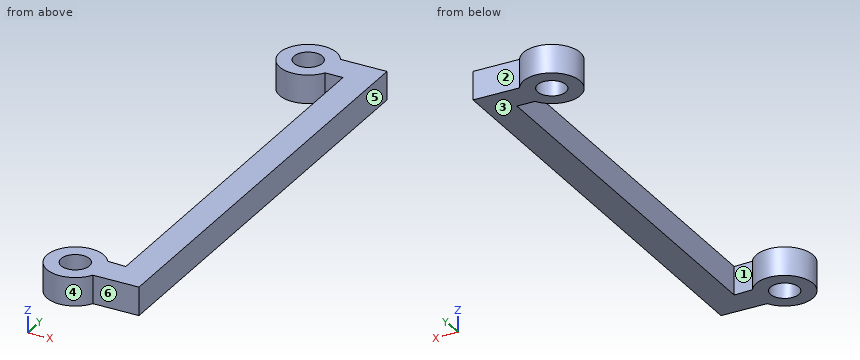
from build123d import *

# Parameters (mm, degrees)
SKETCH_R      = 10
EXTRUDE_DEPTH = 20


with BuildPart() as part:
    # Sketch → Extrude (new body)
    with BuildSketch(Plane.XY):
        with BuildLine():
            Line((11.677619, 0.722876), (24.795086, 0))
            Line((24.795086, 280), (24.795086, 0))
            Line((24.795086, 280), (12.115594, 280))
            ThreePointArc((12.115594, 300), (-25.204914, 290), (12.115594, 280))
            Line((12.115594, 300), (44.795086, 300))
            Line((44.795086, 300), (44.795086, -19.596431))
            Line((44.795086, -19.596431), (12.342408, -19.596431))
            ThreePointArc((11.677619, 0.722876), (-25.194218, -10.653992), (12.342408, -19.596431))
        make_face()
        with Locations((-5.204914, -10)):
            Circle(SKETCH_R, mode=Mode.SUBTRACT)
        with Locations((-5.204914, 290)):
            Circle(SKETCH_R, mode=Mode.SUBTRACT)
    extrude(amount=EXTRUDE_DEPTH)


solid = part.part
The listing builds one solid part. Answer for the finished solid, in the listing's coordinates (mm). Face numbers are marked on the shaded views. A direction names the side the tool comes from. Round coordinates to 2 decimals unless told otherwise and drop trailing zeros. Order: outer loops, then holes, each group sorted by start corner. A loop starts at its lowest first (then second) coordinate and runs counter-clockwise, first axis right, second up. Notation, with made-up numbers: (84, 18.25) - (115, 18.25) arc R22 ccw to (115, 55.25) - close; hole circle Ø11 at (-6, -2). An arc over 180 degrees is marked (long way). Write item = value, one per line. Start each with the question number.
1) Section C-C, the plane x = -2 is taken. Write down the section's boundary in (y, z), plus the area to 3 significant figures.
2) Section D-D, the plane x = 16.5 is taken. Write down the section's boundary in (y, z).
3) For the marked faces 1, 2 and 3, determine the directions among +Z, -Z, +X, -X, +Y, -Y from which every point of the face is accessible in a straight line to the end or side of a thin tool.
4) For a pull along Y with two mould halves and no side action, classify the marked faces 4, 5 and 6 as released by +Y, released by -Y, zero draft, split by the parting line, or undercut.
5) Given pin 1 (8 mm diameter, centred on x = 2, z = 17, fed in from +Y); pin 2 (6 mm diameter, centred on x = -10.5, z = 5.5, fed in from +Y); pin 3 (6 mm diameter, centred on x = 33.5, z = 8, fed in from +Y); pin 4 (12 mm diameter, centred on x = -5.2, y = 290, fed in from +Z), each flat-ended and moving along its own axis, determine where each tip first touches the part or whether it passes through.
6) Straight lines are drawn through the part: L1, parallel to Y at x = -12.5, z = 5; L2, parallel to Y at x = -10, z = 3.5; L3, parallel to X at y = 237, z = 15.25. For each, find the intervals that lie inside material, in ascending order.
7) Section B-B, the plane y = 290 is taken. Write down the section's boundary in (x, z), plus the area to 3 significant figures.
8) Section A-A, the plane z = 3.5 is taken. Write down the section's boundary in (x, y), plus the area to 3 significant figures.
Results list:
q1.outline = (-29.74, 0) - (-19.47, 0) - (-19.47, 20) - (-29.74, 20) - close; (-0.53, 0) - (9.74, 0) - (9.74, 20) - (-0.53, 20) - close; (270.26, 0) - (280.53, 0) - (280.53, 20) - (270.26, 20) - close; (299.47, 0) - (309.74, 0) - (309.74, 20) - (299.47, 20) - close
q1.area = 822 mm^2
q2.outline = (-19.6, 0) - (0.46, 0) - (0.46, 20) - (-19.6, 20) - close; (280, 0) - (300, 0) - (300, 20) - (280, 20) - close
q3.face_1 = +Z, -Z
q3.face_2 = +Z, -Z, +X, +Y
q3.face_3 = -Z, +X, -X, +Y, -Y
q4.face_4 = undercut
q4.face_5 = zero draft
q4.face_6 = released by -Y
q5.pin_1 = 309.74
q5.pin_2 = 309.87
q5.pin_3 = 300
q5.pin_4 = through
q6.L1 = -28.62 to -16.84, -3.16 to 8.62, 271.38 to 283.16, 296.84 to 308.62
q6.L2 = -29.42 to -18.78, -1.22 to 9.42, 270.58 to 281.22, 298.78 to 309.42
q6.L3 = 24.8 to 44.8
q7.outline = (-25.2, 0) - (-15.2, 0) - (-15.2, 20) - (-25.2, 20) - close; (4.8, 0) - (44.8, 0) - (44.8, 20) - (4.8, 20) - close
q7.area = 1,000 mm^2
q8.outline = (11.68, 0.72) arc R20 ccw (long way) to (12.34, -19.6) - (44.8, -19.6) - (44.8, 300) - (12.12, 300) arc R20 ccw (long way) to (12.12, 280) - (24.8, 280) - (24.8, 0) - close; hole circle Ø20 at (-5.2, -10); hole circle Ø20 at (-5.2, 290)
q8.area = 8,710 mm^2
